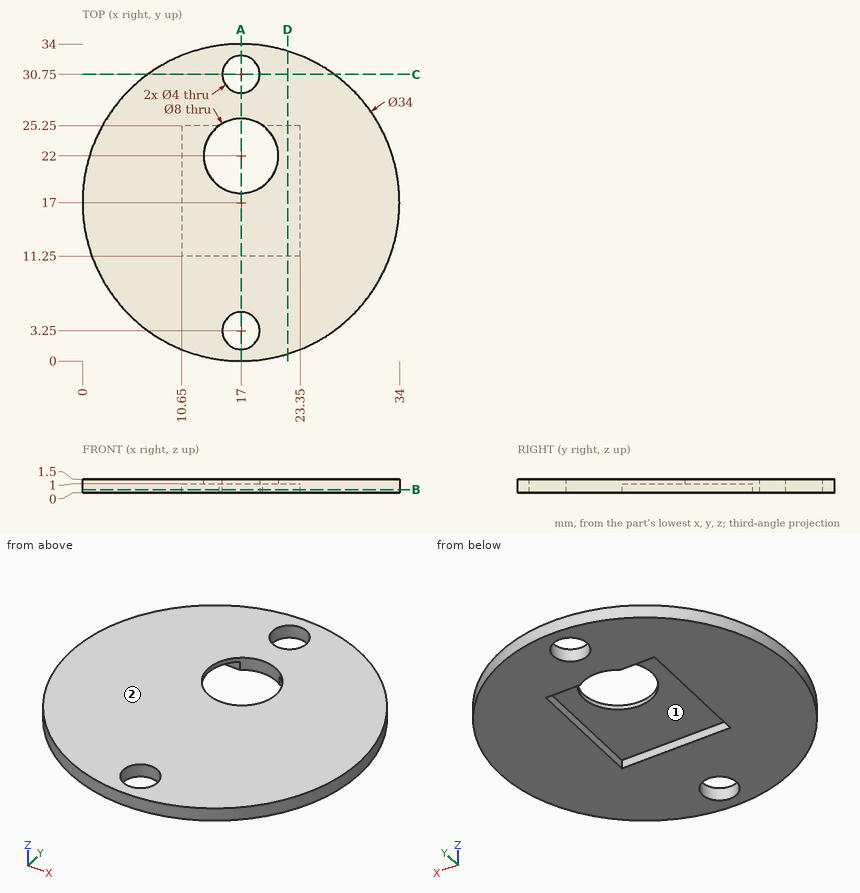
Print and shaded views of the part. All mm, measured from the part's lowest x, y and z. Give positions to 0.01 mm unless a question says otherwise; leave off trailing zeros. Loops run counter-clockwise (first coordinate to the right, second up) from the corner with the lowest first, then second, coordinate; pieces in that order, holes last. Notation, with made-up numbers: (61.25, 72) -> (85.25, 72) arc R4 ccw to (85.25, 76) -> close; hole circle Ø11 at (-20.5, -30). An arc over 180 degrees is marked (long way). Use CSV: the item, a comma, the result in double quotes. Start each with the question number.
1) Slice it at A-A on x = 17. Give the cut face in (y, z).
2) Mould opens along X. For the marked faces 1 and 2 say: released by +X, released by -X, zero draft, split by the parting line, or undercut.
3) Slice it at B-B on z = 0.35. Give the cut face in (x, y), plus the area to 3 significant figures.
4) Slice it at C-C on y = 30.75. Give the cut face in (x, z), plus the area to 3 significant figures.
5) Slice it at D-D on x = 22. Give the cut face in (y, z), plus the area to 3 significant figures.
6) Flat gauge pins, fed straight in: pin 1 Ø0.5 at (x, z) = (21.5, 0.5) entering from -Y; pin 2 Ø0.5 at (y, z) = (16.5, 0.5) entering from +X; pin 3 Ø0.8 at (x, z) = (16, 0.5) entering from +Y. Where does each tip first touch, or does it go through?
7) Wall check: line 1 (Y direction, x = 17, z = 1.15); line 2 (Y direction, x = 17, z = 0.95); line 3 (Y direction, x = 14, z = 0.7). Give the ranges that are in metal, low to high.
Computed values:
1,outline,"(0, 0) -> (1.25, 0) -> (1.25, 1.5) -> (0, 1.5) -> close; (5.25, 0) -> (11.25, 0) -> (11.25, 1) -> (18, 1) -> (18, 1.5) -> (5.25, 1.5) -> close; (26, 0) -> (28.75, 0) -> (28.75, 1.5) -> (26, 1.5) -> close; (32.75, 0) -> (34, 0) -> (34, 1.5) -> (32.75, 1.5) -> close"
2,face 1,"undercut"
2,face 2,"zero draft"
3,outline,"circle Ø34 at (17, 17); hole (10.65, 11.25) -> (23.35, 11.25) -> (23.35, 25.25) -> (19.33, 25.25) arc R4 ccw to (14.67, 25.25) -> (10.65, 25.25) -> close; hole circle Ø4 at (17, 3.25); hole circle Ø4 at (17, 30.75)"
3,area,"703 mm^2"
4,outline,"(7, 0) -> (15, 0) -> (15, 1.5) -> (7, 1.5) -> close; (19, 0) -> (27, 0) -> (27, 1.5) -> (19, 1.5) -> close"
4,area,"24.0 mm^2"
5,outline,"(0.75, 0) -> (11.25, 0) -> (11.25, 1) -> (25.25, 1) -> (25.25, 0) -> (33.25, 0) -> (33.25, 1.5) -> (0.75, 1.5) -> close"
5,area,"34.7 mm^2"
6,pin 1,"stops at y = 0.54"
6,pin 2,"stops at x = 34"
6,pin 3,"stops at y = 33.99"
7,line 1,"y = 0 to 1.25, 5.25 to 18, 26 to 28.75, 32.75 to 34"
7,line 2,"y = 0 to 1.25, 5.25 to 11.25, 26 to 28.75, 32.75 to 34"
7,line 3,"y = 0.27 to 11.25, 25.25 to 33.73"
